The model under review builds one solid part; all positions refer to its coordinate system, in mm. A direction names the side the tool comes from. Coordinates: 2 decimals unless noted, no trailing zeros. Order: outer loops, then holes, each group sorted by start corner. A loop starts at its lowest first (then second) coordinate and runs counter-clockwise, first axis right, second up.
```python
from build123d import *

# Parameters (mm, degrees)
SKETCH_1_W         = 32
SKETCH_1_H         = 30
SKETCH_1_R         = 1.6
EXTRUDE_1_DEPTH    = 4
SKETCH2_W          = 17
SKETCH2_H          = 5
CUT_EXTRUDE2_DEPTH = 5


with BuildPart() as part:
    # Эскиз1 → Бобышка-Вытянуть1 (new body)
    with BuildSketch(Plane(origin=(15.473923778, 0, 0), x_dir=(0, 0, -1), z_dir=(1, 0, 0))):
        with Locations((2.763696673, 23.493617857)):
            Rectangle(SKETCH_1_W, SKETCH_1_H)
        with Locations((-7.236303327, 31.493617857)):
            Circle(SKETCH_1_R, mode=Mode.SUBTRACT)
        with Locations((12.763696673, 31.493617857)):
            Circle(SKETCH_1_R, mode=Mode.SUBTRACT)
        with Locations((-7.236303327, 15.493617857)):
            Circle(SKETCH_1_R, mode=Mode.SUBTRACT)
        with Locations((12.763696673, 15.493617857)):
            Circle(SKETCH_1_R, mode=Mode.SUBTRACT)
    extrude(amount=EXTRUDE_1_DEPTH)

    # Sketch2 → Cut-Extrude2 (cut, through all)
    with BuildSketch(Plane.ZY.offset(-15.473923778)):
        with Locations((-2.763696673, 23.493617857)):
            Rectangle(SKETCH2_W, SKETCH2_H)
    extrude(amount=-CUT_EXTRUDE2_DEPTH, mode=Mode.SUBTRACT)


solid = part.part
```
(1) We need section A-A, the plane y = 22. Write out the cut boundary in (x, z), and give its area (3 significant figures).
A:
outline: (15.47, -18.76) - (19.47, -18.76) - (19.47, -11.26) - (15.47, -11.26) - close; (15.47, 5.74) - (19.47, 5.74) - (19.47, 13.24) - (15.47, 13.24) - close
area: 60.0 mm2
(2) Draft analysis for pull direction Y (two halves, no side actions). For faces 1 (the face through (17, 8.494, -3)), 2 (the face through (19.474, 20, -3)), 3 (the face through (17.446, 30.52, 8.506)), state which applies: released by +Y, released by -Y, zero draft, split by the parting line, or undercut.
A:
face 1: released by -Y
face 2: zero draft
face 3: undercut
(3) Wall thickness on probe 1 along Z at (x, y) = (19.1, 22); probe 2 along Y at (x, z) = (17.8, -6); probe 3 along Y at (x, z) = (18.15, 6.5): over which ranges is each line inside the solid? List them lowest first.
A:
probe 1: z = -18.76 to -11.26, 5.74 to 13.24
probe 2: y = 8.49 to 20.99, 25.99 to 38.49
probe 3: y = 8.49 to 14.07, 16.91 to 30.07, 32.91 to 38.49
(4) We need section B-B, the plane z = 4. Write out the cut boundary in (x, y), and give its area (3 significant figures).
A:
outline: (15.47, 8.49) - (19.47, 8.49) - (19.47, 20.99) - (15.47, 20.99) - close; (15.47, 25.99) - (19.47, 25.99) - (19.47, 38.49) - (15.47, 38.49) - close
area: 100 mm2
(5) We need section D-D, the plane y = 32.5. Write out the cut boundary in (x, z).
A:
outline: (15.47, -18.76) - (19.47, -18.76) - (19.47, -14.01) - (15.47, -14.01) - close; (15.47, -11.52) - (19.47, -11.52) - (19.47, 5.99) - (15.47, 5.99) - close; (15.47, 8.48) - (19.47, 8.48) - (19.47, 13.24) - (15.47, 13.24) - close
(6) Machinability: for faces 4 (the face through (17, 20.994, -3)), 5 (the face through (17, 23, -18.764)), which of the approach directions +Z, -Z, +X, -X, +Y, -Y give a long, thin tool a straight path to every point of the face, cutting with its end or side? Answer none if there is none.
A:
face 4: +X, -X
face 5: -Z, +X, -X, +Y, -Y
(7) We need section C-C, the plane x = 19.1. Write out the cut boundary in (y, z), and give its area (3 significant figures).
A:
outline: (8.49, -18.76) - (38.49, -18.76) - (38.49, 13.24) - (8.49, 13.24) - close; hole circle Ø3.2 at (15.49, -12.76); hole circle Ø3.2 at (15.49, 7.24); hole (20.99, -11.26) - (25.99, -11.26) - (25.99, 5.74) - (20.99, 5.74) - close; hole circle Ø3.2 at (31.49, -12.76); hole circle Ø3.2 at (31.49, 7.24)
area: 843 mm2
